The model under review builds one solid part; all positions refer to its coordinate system, in mm. Coordinates: 2 decimals unless noted, no trailing zeros. Write each loop counter-clockwise with the first axis right and the second up, starting at its lowest first coordinate (ties: lowest second). Pieces come first, ordered by that corner, then holes.
1) Add section D-D, the plane y = 8. State the section outline as (x, z) points.
2) Add section A-A, the plane y = -47. State the section outline as (x, z) points, then the cut area to 3 significant figures.
3) For line 1 (Y direction, x = 43, z = 1.6); line 2 (Y direction, x = 15, z = 2.75); line 3 (Y direction, x = -5.75, z = 0.95), list the stretches that pass through material, from the lowest coordinate up.
4) For P1, Ø1.5, axis at y = -4, z = 2, coming from the -X side; P2, Ø1.3, axis at y = -12.5, z = 1.5, coming from the -X side; P3, Ø1.8, axis at x = 15.75, y = 8, coming from the -Z side; P4, Ø1, axis at x = 29, z = 1, coming from the +Y side, all flat-tipped, find the tip position at first contact; note any pin that passes through.
5) Add section B-B, the plane x = 59. State the section outline as (y, z) points, then the cut area to 3 significant figures.
6) Add section C-C, the plane x = 10.25. State the section outline as (y, z) points, then the cut area to 3 significant figures.
from build123d import *

# Parameters (mm, degrees)
BOSS_EXTRU_1_DEPTH      = 3
D_GAGEMENT_M21_D        = 3
CHANFREIN1_SIZE         = 1.5
CHANFREIN2_SIZE         = 6
CHANFREIN2_SIZE2        = 3
CONG_1_R                = 2
CONG_2_R                = 10
CONG_2_2_R              = 5
CONG_3_R                = 0.8
D_GAGEMENT_M31_D        = 3.4
ENL_V_MAT_EXTRU_1_REACH = 5
FILLET_1_R              = 3
FILLET_2_R              = 1
SKETCH_5_R              = 1.5
CUT_EXTRUDE_2_DEPTH     = 3
SKETCH_6_R              = 1.5
EXTRUDE_3_DEPTH         = 3


with BuildPart() as part:
    # Esquisse1 → Boss.-Extru.1 (new body)
    with BuildSketch(Plane.XY):
        Polygon((48.900602827, -4.024), (19.677471167, 17), (-17.75, 17), (-17.75, 10.3), (12.55, 10.3), (12.55, -10.3), (-9.75, -10.3), (-9.75, -16), (19.295179393, -24.993298238), (46.71123265, -66.806693506), (46.285412403, -78.306693506), (62.357629227, -91.032016541), (72.595795313, -84.772627178), (67.901253291, -77.094002614), align=None)
        Polygon((28.816069815, -26.747772307), (44.278044238, -14.062058021), (55.602935243, -57.613715208), (51.023072953, -60.616622474), align=None, mode=Mode.SUBTRACT)
        Polygon((23.25, -19.026221012), (23.25, 5.973778988), (39.485073144, -5.706221012), align=None, mode=Mode.SUBTRACT)
    extrude(amount=BOSS_EXTRU_1_DEPTH)

    # D_gagement M21 (through all)
    with Locations(Plane.XY.offset(3)):
        with Locations((-13.75, 13.5), (-5.75, 13.5), (2.25, 13.5), (10.25, 13.5), (15.75, 8), (15.75, -8), (10.25, -13.5)):
            Hole(D_GAGEMENT_M21_D / 2)

    # Chanfrein1
    chanfrein1_edges = [part.edges().sort_by_distance(p)[0] for p in [
        (-17.75, 10.3, 1.5),
    ]]
    chamfer(chanfrein1_edges, length=CHANFREIN1_SIZE)

    # Chanfrein2
    chanfrein2_edges = [part.edges().sort_by_distance(p)[0] for p in [
        (-17.75, 17, 1.5),
    ]]
    chanfrein2_side = [part.faces().sort_by_distance(p)[0] for p in [
        (0.963735584, 17, 1.5),
    ]]
    chamfer(chanfrein2_edges, length=CHANFREIN2_SIZE, length2=CHANFREIN2_SIZE2, reference=chanfrein2_side[0])

    # Cong_1
    cong_1_edges = [part.edges().sort_by_distance(p)[0] for p in [
        (72.595795313, -84.772627178, 1.5),
        (62.357629227, -91.032016541, 1.5),
        (23.25, 5.973778988, 1.5),
        (23.25, -19.026221012, 1.5),
        (39.485073144, -5.706221012, 1.5),
        (51.023072953, -60.616622474, 1.5),
        (55.602935243, -57.613715208, 1.5),
        (44.278044238, -14.062058021, 1.5),
        (28.816069815, -26.747772307, 1.5),
    ]]
    fillet(cong_1_edges, radius=CONG_1_R)

    # Cong_2
    cong_2_edges = [part.edges().sort_by_distance(p)[0] for p in [
        (19.677471167, 17, 1.5),
        (48.900602827, -4.024, 1.5),
        (19.295179393, -24.993298238, 1.5),
        (46.71123265, -66.806693506, 1.5),
        (67.901253291, -77.094002614, 1.5),
    ]]
    fillet(cong_2_edges, radius=CONG_2_R)

    # Cong_2 2
    cong_2_2_edges = [part.edges().sort_by_distance(p)[0] for p in [
        (46.285412403, -78.306693506, 1.5),
    ]]
    fillet(cong_2_2_edges, radius=CONG_2_2_R)

    # Cong_3
    cong_3_edges = [part.edges().sort_by_distance(p)[0] for p in [
        (-9.75, -10.3, 1.5),
        (12.55, -10.3, 1.5),
        (12.55, 10.3, 1.5),
    ]]
    fillet(cong_3_edges, radius=CONG_3_R)

    # D_gagement M31 (through all)
    with Locations(Plane(origin=(0, 0, 0), x_dir=(-1, 0, 0), z_dir=(0, 0, -1))):
        with Locations((-44, -8.146072926), (-59, -61.892892977), (-51.375748619, -75.959548261)):
            Hole(D_GAGEMENT_M31_D / 2)

    # Esquisse6 → Enl_v. mat.-Extru.1 (cut, up to next)
    with BuildSketch(Plane.XY.offset(3), mode=Mode.PRIVATE) as enl_v_mat_extru_1_sk1:
        Polygon((50.923621455, -68.720394376), (56.895885005, -65.069083914), (62.112042808, -73.600888985), (56.139779258, -77.252199447), align=None)
    enl_v_mat_extru_1_tool1 = extrude(enl_v_mat_extru_1_sk1.sketch, amount=-ENL_V_MAT_EXTRU_1_REACH, mode=Mode.PRIVATE) & part.part
    add(enl_v_mat_extru_1_tool1.solids().sort_by_distance((56.517832, -71.160642, 3))[0], mode=Mode.SUBTRACT)

    # Fillet 1
    fillet_1_edges = [part.edges().sort_by_distance(p)[0] for p in [
        (-9.75, -16, 1.5),
    ]]
    fillet(fillet_1_edges, radius=FILLET_1_R)

    # Fillet 2
    fillet_2_edges = [part.edges().sort_by_distance(p)[0] for p in [
        (-17.75, 14, 1.5),
        (-11.75, 17, 1.5),
    ]]
    fillet(fillet_2_edges, radius=FILLET_2_R)

    # Sketch 5 → Cut-Extrude 2 (cut)
    with BuildSketch(Plane(origin=(0, 0, 0), x_dir=(-1, 0, 0), z_dir=(0, 0, -1))):
        with Locations((5.75, -13.5)):
            Circle(SKETCH_5_R)
    extrude(amount=-CUT_EXTRUDE_2_DEPTH, mode=Mode.SUBTRACT)

    # Sketch 6 → Extrude 3 (add)
    with BuildSketch(Plane(origin=(0, 0, 0), x_dir=(-1, 0, 0), z_dir=(0, 0, -1))):
        with Locations((13.75, 13.5)):
            Circle(SKETCH_6_R)
        with Locations((-2.25, 13.5)):
            Circle(SKETCH_6_R)
    extrude(amount=-EXTRUDE_3_DEPTH)


solid = part.part
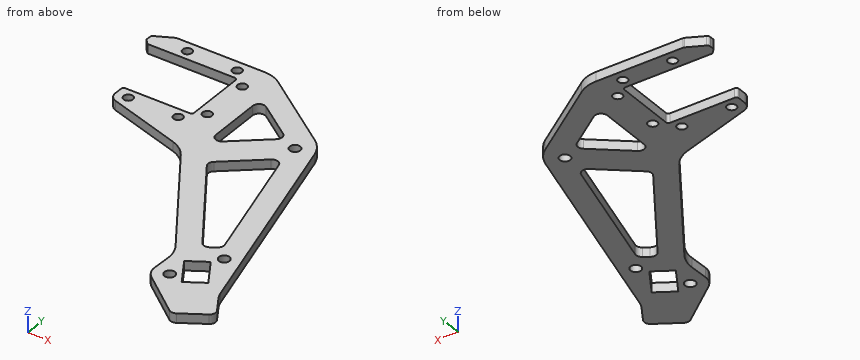
Geometry results:
1. outline: (12.55, 0) - (14.25, 0) - (14.25, 3) - (12.55, 3) - close; (17.25, 0) - (32.19, 0) - (32.19, 3) - (17.25, 3) - close
2. outline: (33.72, 0) - (42.09, 0) - (42.09, 3) - (33.72, 3) - close; (52.84, 0) - (60.08, 0) - (60.08, 3) - (52.84, 3) - close
2. area: 46.8 mm2
3. line 1: y = -61.15 to -48.38, -15.6 to -9.52, -6.77 to 0.22
3. line 2: y = -23.66 to -9.3, -6.7 to 6.7, 9.3 to 17
3. line 3: y = -17.24 to -15, -12 to -10.3, 10.3 to 12, 15 to 17
4. P1: stops at x = 12.55
4. P2: stops at x = -9.75
4. P3: passes through
4. P4: stops at y = 10.65
5. outline: (-88.37, 0) - (-75.5, 0) - (-75.5, 3) - (-88.37, 3) - close; (-68.51, 0) - (-63.59, 0) - (-63.59, 3) - (-68.51, 3) - close; (-60.19, 0) - (-42.86, 0) - (-42.86, 3) - (-60.19, 3) - close
5. area: 105 mm2
6. outline: (-22.19, 0) - (-15, 0) - (-15, 3) - (-22.19, 3) - close; (-12, 0) - (-10.3, 0) - (-10.3, 3) - (-12, 3) - close; (10.3, 0) - (12, 0) - (12, 3) - (10.3, 3) - close; (15, 0) - (17, 0) - (17, 3) - (15, 3) - close
6. area: 37.8 mm2
